Part model, mm, in its own coordinate system. Face numbers are marked on the shaded views. A direction names the side the tool comes from. Give positions to 0.01 mm unless a question says otherwise; leave off trailing zeros. Order: outer loops, then holes, each group sorted by start corner. A loop starts at its lowest first (then second) coordinate and runs counter-clockwise, first axis right, second up. Notation, with made-up numbers: (20.25, 35) - (24.25, 35) arc R20 cw to (24.25, 74) - close; hole circle Ø9 at (-8, 83.5). An arc over 180 degrees is marked (long way). One line per item, written item: value.
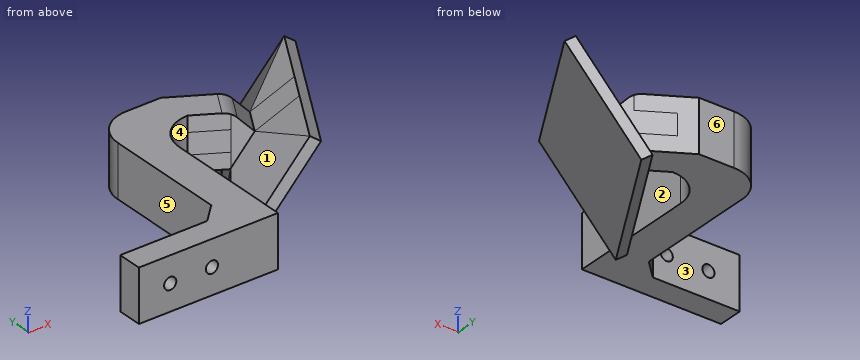
```python
from build123d import *

# Parameters (mm, degrees)
SKETCH_1_W               = 40
SKETCH_1_H               = 15
EXTRUDE_1_DEPTH          = 7
SKETCH_3_W               = 10
SKETCH_3_H               = 6
EXTRUDE_2_DEPTH          = 50
EXTRUDE_5_DEPTH          = 6
FILLET_1_R               = 10
SKETCH_7_R               = 1.75
CUT_EXTRUDE_3_DEPTH      = 10
SKETCH_16_W              = 6
SKETCH_16_H              = 8.660254038
EXTRUDE_11_DEPTH         = 10
EXTRUDE_12_DEPTH         = 8.66
EXTRUDE_14_DEPTH         = 3
EXTRUDE_15_DEPTH         = 4.5
EXTRUDE_15_DEPTH_BACK    = 10.5
EXTRUDE_17_DEPTH         = 8.66
EXTRUDE_22_DEPTH         = 8.66
EXTRUDE_23_DEPTH         = 15
FILLET_2_R               = 10
EXTRUDE_24_DEPTH         = 35
CUT_EXTRUDE_4_DEPTH      = 35
CUT_EXTRUDE_4_DEPTH_BACK = 35
CUT_EXTRUDE_5_DEPTH      = 35
CUT_EXTRUDE_5_DEPTH_BACK = 35
FILLET_3_R               = 5


with BuildPart() as part:
    # 草图1 → 凸台-拉伸1 (new body)
    with BuildSketch(Plane(origin=(0, 0, 0), x_dir=(1, 0, 0), z_dir=(0, 1, 0))):
        with Locations((-15, 0)):
            Rectangle(SKETCH_1_W, SKETCH_1_H)
    extrude(amount=EXTRUDE_1_DEPTH)

    # 草图3 → 凸台-拉伸2 (add)
    with BuildSketch(Plane(origin=(0, 7, 0), x_dir=(1, 0, 0), z_dir=(0, 1, 0))):
        Rectangle(SKETCH_3_W, SKETCH_3_H)
    extrude(amount=EXTRUDE_2_DEPTH)

    # 草图4 → 凸台-拉伸5 (add)
    with BuildSketch(Plane.XY.offset(3)):
        Polygon((5, 57), (5, 47), (15, 47), (19.330127019, 54.5), (15, 57), align=None)
    extrude(amount=-EXTRUDE_5_DEPTH)

    # 圆角1
    fillet_1_edges = [part.edges().sort_by_distance(p)[0] for p in [
        (-5, 57, 0),
    ]]
    fillet(fillet_1_edges, radius=FILLET_1_R)

    # 草图7 → 切除-拉伸3 (cut)
    with BuildSketch(Plane(origin=(0, 7, 0), x_dir=(1, 0, 0), z_dir=(0, 1, 0))):
        with Locations(Location((-26, 0, 0), (0, 0, 270))):
            Circle(SKETCH_7_R)
        with Locations(Location((-14, 0, 0), (0, 0, 270))):
            Circle(SKETCH_7_R)
    extrude(amount=-CUT_EXTRUDE_3_DEPTH, mode=Mode.SUBTRACT)

    # 草图16 → 凸台-拉伸11 (add)
    with BuildSketch(Plane(origin=(-9.101596989, 5.254809472, 0), x_dir=(0, 0, -1), z_dir=(0.8660254037844403, -0.4999999999999973, 0))):
        with Locations((0, 52.533320997)):
            Rectangle(SKETCH_16_W, SKETCH_16_H)
    extrude(amount=EXTRUDE_11_DEPTH)

    # 草图17 → 凸台-拉伸12 (add)
    with BuildSketch(Plane(origin=(28.431724008, 49.245190528, 0), x_dir=(0.8660254037844402, -0.4999999999999975, 0), z_dir=(0.4999999999999975, 0.8660254037844402, 0))):
        Polygon((-0.509618943, -3), (6.561448869, 4.071067812), (4.387416664, 7.7860808), (-0.509618943, 3), align=None)
    extrude(amount=-EXTRUDE_12_DEPTH)

    # 草图19 → 凸台-拉伸14 (add)
    with BuildSketch(Plane(origin=(5.769699285, -3.331137436, -3.898775098), x_dir=(-0.6556667796433489, -0.35687658637483116, -0.6653872377567577), z_dir=(0.7474459160042376, -0.43153810080973004, -0.5050737274875003))):
        Polygon((-33.928130068, 69.297295246), (-5.267738986, 34.604616147), (-32.250933841, 12.313200861), (-60.911324922, 47.00587996), align=None)
    extrude(amount=EXTRUDE_14_DEPTH)

    # 草图20 → 凸台-拉伸15 (add, two sides: drawn at the far end of the back side and taken through both)
    with BuildSketch(Plane(origin=(0, 0, -3), x_dir=(-1, 0, 0), z_dir=(0, 0, -1)).offset(-EXTRUDE_15_DEPTH_BACK)):
        with BuildLine():
            Line((-5, 7), (5, 7))
            Line((5, 7), (5, 47))
            ThreePointArc((5, 47), (2.071067812, 54.071067812), (-5, 57))
            Line((-5, 57), (-15, 57))
            Line((-15, 57), (-27.990381057, 49.5))
            Line((-27.990381057, 49.5), (-23.660381057, 42.000220003))
            Line((-23.660381057, 42.000220003), (-15, 47))
            Line((-15, 47), (-5, 47))
            Line((-5, 47), (-5, 7))
        make_face()
    extrude(amount=EXTRUDE_15_DEPTH + EXTRUDE_15_DEPTH_BACK)

    # 草图21 → 凸台-拉伸17 (add)
    with BuildSketch(Plane(origin=(28.431724008, 49.245190528, 0), x_dir=(0.8660254037844402, -0.4999999999999975, 0), z_dir=(0.4999999999999975, 0.8660254037844402, 0))):
        Polygon((-0.509618943, 7.5), (-0.509618943, 3), (4.387416664, 7.7860808), align=None)
        Polygon((-0.509618943, -7.5), (8.29635004, 1.106447339), (6.561448869, 4.071067812), (-0.509618943, -3), align=None)
    extrude(amount=-EXTRUDE_17_DEPTH)

    # 草图22 → 凸台-拉伸22 (add)
    with BuildSketch(Plane(origin=(28.431724008, 49.245190528, 0), x_dir=(0.8660254037844402, -0.4999999999999975, 0), z_dir=(0.4999999999999975, 0.8660254037844402, 0))):
        Polygon((4.387416664, 7.7860808), (-2.41816344, 19.41553984), (-0.509618943, 7.5), align=None)
        Polygon((8.29635004, 1.106447339), (15.259417022, -10.792127217), (4.967687183, -2.146796188), align=None)
    extrude(amount=-EXTRUDE_22_DEPTH)

    # 草图23 → 凸台-拉伸23 (add)
    with BuildSketch(Plane.XY.offset(7.5)):
        Polygon((-5, 7), (-10, 7), (-5, 12), align=None)
    extrude(amount=-EXTRUDE_23_DEPTH)

    # 圆角2
    fillet_2_edges = [part.edges().sort_by_distance(p)[0] for p in [
        (5, 47, 0),
    ]]
    fillet(fillet_2_edges, radius=FILLET_2_R - 0.0001)  # a hair under: the kernel refuses the full size


with BuildPart() as extrude_24_tool:
    # 草图24 → 凸台-拉伸24 (new body)
    with BuildSketch(Plane(origin=(7.445343505, -4.298571076, 14.690902319), x_dir=(0.8992638085264243, 0.12283526789294275, -0.4198048351748937), z_dir=(0.43740667881795164, -0.25253686369234724, 0.8630762016194644))):
        Polygon((34.27908934, 45.482482988), (38.032691816, 42.971530425), (48.135364869, 58.073933853), align=None)
        Polygon((29.464039564, 38.284504407), (33.21764204, 35.773551844), (23.114898365, 20.671042842), align=None)
    extrude(amount=-EXTRUDE_24_DEPTH)


with BuildPart() as part_1:
    add(part.part)


with BuildPart() as part_2:
    # 凸台-拉伸24: joined with extrude_24_tool
    add(part_1.part.fuse(extrude_24_tool.part, tol=0.00001))

    # 草图25 → 切除-拉伸4 (cut, two sides: drawn at the far end of the back side and taken through both)
    with BuildSketch(Plane(origin=(28.431724014, 49.245190525, -8e-09), x_dir=(0.866025403727626, -0.5000000000984025, 7.809544934800217e-11), z_dir=(-0.5000000000984025, -0.866025403727626, 1.35265286075167e-10)).offset(-CUT_EXTRUDE_4_DEPTH_BACK)):
        Polygon((11.361749763, 13.073049031), (15.259417021, 10.792127222), (4.967687177, 2.146796194), align=None)
    extrude(amount=CUT_EXTRUDE_4_DEPTH + CUT_EXTRUDE_4_DEPTH_BACK, mode=Mode.SUBTRACT)

    # 草图26 → 切除-拉伸5 (cut, two sides: drawn at the far end of the back side and taken through both)
    with BuildSketch(Plane(origin=(24.101724013, 41.745410529, -7e-09), x_dir=(0.8660254037276265, -0.5000000000984015, 7.809507734629167e-11), z_dir=(0.5000000000984015, 0.8660254037276265, -1.3526464174930455e-10)).offset(-CUT_EXTRUDE_5_DEPTH_BACK)):
        Polygon((-0.677635102, 7.499999992), (-2.41816345, 19.415539829), (-6.315830703, 17.134618023), align=None)
    extrude(amount=CUT_EXTRUDE_5_DEPTH + CUT_EXTRUDE_5_DEPTH_BACK, mode=Mode.SUBTRACT)

    # 圆角3
    fillet_3_edges = [part_2.edges().sort_by_distance(p)[0] for p in [
        (25.825381057, 45.750110002, 7.5),
    ]]
    fillet(fillet_3_edges, radius=FILLET_3_R)


solid = part_2.part
```
1) Pin check, flat tips, straight feed: pin 1 (16.5 mm diameter, centred on x = -22.5, z = 3.5, fed in from +Y); pin 2 (5.5 mm diameter, centred on x = 21.5, y = 45, fed in from -Z); pin 3 (1.5 mm diameter, centred on y = 30, z = -7.5, fed in from +X). Stop position of each tip, or through.
Outcome:
pin 1: stops at y = 7
pin 2: stops at z = -20.17
pin 3: stops at x = 27.26
2) Cut at C-C, the plane z = 0. Give the number of separate pieces and of enclosed holes in the cut face, then the cut area to 3 significant figures.
Outcome:
separate pieces: 3
enclosed holes: 0
area: 1,290 mm^2
3) Mould opens along X. For the marked faces 4, 5 and 6 say: released by +X, released by -X, zero draft, split by the parting line, or undercut.
Outcome:
face 4: undercut
face 5: released by -X
face 6: zero draft
4) Cut at D-D, the plane y = 6. Give the cut face in (x, z), then the cut area to 3 significant figures.
Outcome:
outline: (-35, -7.5) - (5, -7.5) - (5, 7.5) - (-35, 7.5) - close; hole circle Ø3.5 at (-26, 0); hole circle Ø3.5 at (-14, 0)
area: 581 mm^2
5) Cut at A-A, the plane x = -14. Give the cut face in (y, z).
Outcome:
outline: (0, -7.5) - (7, -7.5) - (7, -1.75) - (0, -1.75) - close; (0, 1.75) - (7, 1.75) - (7, 7.5) - (0, 7.5) - close
6) Which spindle directions (+Z, -Z, +X, -X, +Y, -Y) get a long thin tool onto all of the face, cutting with end or side? Do the marked faces 1, 2 and 3. Say none if no direction does.
Outcome:
face 1: +Z
face 2: +Z, -Z, -Y
face 3: +Z, -Z, -X, +Y
7) Drill centre lines: line 1 along X through (y, z) = (4, 0); line 2 along Y through (x, z) = (-10, 7); line 3 along X through (y, z) = (5.5, 1). Where is each one in solid material? Low to high. Write a range as from..to.
Outcome:
line 1: x = -35..-27.75, -24.25..-15.75, -12.25..5
line 2: y = 0..7
line 3: x = -35..-27.44, -24.56..-15.44, -12.56..5
8) Cut at B-B, the plane y = 32.5. Give the cut face in (x, z), then the cut area to 3 significant figures.
Outcome:
outline: (-5, -7.5) - (5, -7.5) - (5, 7.5) - (-5, 7.5) - close; (15.97, -19.42) - (18.96, -20.93) - (39.37, 9.28) - (36.38, 10.79) - (28.35, 4.95) - (16.69, -15.18) - close
area: 350 mm^2
